Read the model definition and answer for the solid it produces. Units are mm, in the model's axes. A direction names the side the tool comes from. Give positions to 0.01 mm unless a question says otherwise; leave off trailing zeros. Order: outer loops, then holes, each group sorted by start corner. A loop starts at its lowest first (then second) coordinate and runs counter-clockwise, first axis right, second up. Notation, with made-up numbers: (-25.75, -19) - (22.25, -19) arc R20 cw to (22.25, 20) - close; hole circle Ø7 at (-26.75, -15.5). An arc over 180 degrees is marked (long way). Write each question's results on one line, items separated by ' | '.
from build123d import *

# Parameters (mm, degrees)
SKETCH_1_R                  = 22
EXTRUDE_1_DEPTH             = 18
SKETCH_2_W                  = 10
SKETCH_2_H                  = 12
EXTRUDE_2_DEPTH             = 22
SKETCH_3_W                  = 15
SKETCH_3_H                  = 12
EXTRUDE_3_DEPTH             = 2
EXTRUDE_3_DIRECTION_2_REACH = 43.195


with BuildPart() as part:
    # 草图1 → 凸台-拉伸1 (new body)
    with BuildSketch(Plane(origin=(0, 0, 0), x_dir=(1, 0, 0), z_dir=(0, 1, 0))):
        with Locations(Location((0, 0, 0), (0, 0, 270))):
            Circle(SKETCH_1_R)
    extrude(amount=EXTRUDE_1_DEPTH)

    # 草图2 → 凸台-拉伸2 (add)
    with BuildSketch(Plane.XZ):
        Rectangle(SKETCH_2_W, SKETCH_2_H)
    extrude(amount=EXTRUDE_2_DEPTH)

    # 草图3 → 凸台-拉伸3 (add)
    with BuildSketch(Plane(origin=(5, 0, 0), x_dir=(0, 0, -1), z_dir=(1, 0, 0))):
        with Locations((0, -13)):
            Rectangle(SKETCH_3_W, SKETCH_3_H)
    extrude(amount=EXTRUDE_3_DEPTH)

    # 凸台-拉伸3 direction 2: up to this face of the body (flat: up to its plane)
    extrude_3_direction_2_end = Plane(part.part.faces().sort_by_distance((-5, -11, 0))[0])
    # 草图3 → 凸台-拉伸3 direction 2 (add, up to the picked face)
    with BuildSketch(Plane(origin=(5, 0, 0), x_dir=(0, 0, -1), z_dir=(1, 0, 0)), mode=Mode.PRIVATE) as extrude_3_direction_2_sk1:
        with Locations((0, -13)):
            Rectangle(SKETCH_3_W, SKETCH_3_H)
    extrude_3_direction_2_tool1 = split(extrude(extrude_3_direction_2_sk1.sketch, amount=-EXTRUDE_3_DIRECTION_2_REACH, mode=Mode.PRIVATE), bisect_by=extrude_3_direction_2_end, keep=Keep.BOTH, mode=Mode.PRIVATE)
    add(extrude_3_direction_2_tool1.solids().sort_by(Axis((5, -13, 0), (-1, 0, 0)))[0])


solid = part.part
(1) For faces 4 (the face through (1, -13, 7.5)), 5 (the face through (-5, -11, 0)), 6 (the face through (5, -3, 0)), 7 (the face through (1, -13, -7.5)), 8 (the face through (7, -13, 0)), determine the directions among +Z, -Z, +X, -X, +Y, -Y from which every point of the face is accessible in a straight line to the end or side of a thin tool.
Conclusion:
face 4: +Z, +X, -X, -Y | face 5: +Z, -Z, -X, -Y | face 6: +Z, -Z, +X | face 7: -Z, +X, -X, -Y | face 8: +Z, -Z, +X, -Y
(2) Section C-C (y = -13.5) is taken. Give the vertices of the cut face in (x, z), plus the area to 3 significant figures.
Conclusion:
outline: (-5, -7.5) - (7, -7.5) - (7, 7.5) - (-5, 7.5) - close | area: 180 mm^2
(3) Section B-B (x = 0) is taken. Give the vertices of the cut face in (y, z), plus the area to 3 significant figures.
Conclusion:
outline: (-22, -6) - (-19, -6) - (-19, -7.5) - (-7, -7.5) - (-7, -6) - (0, -6) - (0, -22) - (18, -22) - (18, 22) - (0, 22) - (0, 6) - (-7, 6) - (-7, 7.5) - (-19, 7.5) - (-19, 6) - (-22, 6) - close | area: 1,090 mm^2
(4) Section A-A (z = 0) is taken. Give the vertices of the cut face in (x, y), plus the area to 3 significant figures.
Conclusion:
outline: (-22, 0) - (-5, 0) - (-5, -22) - (5, -22) - (5, -19) - (7, -19) - (7, -7) - (5, -7) - (5, 0) - (22, 0) - (22, 18) - (-22, 18) - close | area: 1,040 mm^2
(5) Section D-D (y = 1) is taken. Give the vertices of the cut face in (x, z).
Conclusion:
outline: circle Ø44 at (0, 0)
(6) The mould has two halves that part along Y. Classify faces 1 (the face through (0, -20, 6)), 2 (the face through (0, -3, 6)), 3 (the face through (0, 18, 0)): pulls with the +Y half, pulls with the -Y half, needs draft (parallel to the pull), parting line crosses it, or undercut.
Conclusion:
face 1: needs draft | face 2: undercut | face 3: pulls with the +Y half
(7) Each of these flat-tipped pins is pushed along its axis until it touches: pin 1 (3.5 mm diameter, centred on y = -5, z = 0.5, fed in from +X); pin 2 (9.5 mm diameter, centred on x = -1.5, y = -13, fed in from -Z); pin 3 (1.5 mm diameter, centred on x = -1.5, y = -20, fed in from +Z); pin 4 (6 mm diameter, centred on x = 11, y = -16.5, fed in from -Z). Where does it stop, or does it pass through?
Conclusion:
pin 1: x = 5 | pin 2: z = -7.5 | pin 3: z = 6 | pin 4: through
(8) Consider probe 1 along Y at (x, z) = (0, 7); probe 2 along Z at (x, y) = (-2, -17); probe 3 along Y at (x, z) = (4.5, 16). Determine where each line is inside the solid, lowest interval first. Write a range as [from, to].
Conclusion:
probe 1: [-19, -7], [0, 18] | probe 2: [-7.5, 7.5] | probe 3: [0, 18]
